Autodesk Inventor part; units mm, degrees
ref_plane "YZ Plane" through (0, 0, 0) normal (1, 0, 0) x (0, 1, 0)
ref_plane "XZ Plane" through (0, 0, 0) normal (0, 1, 0) x (-1, 0, 0)
ref_plane "XY Plane" through (0, 0, 0) normal (0, 0, 1) x (1, 0, 0)
sketch "Sketch1" plane through (0, 0, 0) normal (0, 0, 1) x (1, 0, 0)
  line L0 (-20.5, -12.375) -> (20.5, -12.375)
  line L1 (20.5, -12.375) -> (20.5, 12.375)
  line L2 (20.5, 12.375) -> (-20.5, 12.375)
  line L3 (-20.5, 12.375) -> (-20.5, -12.375)
  line L4 (-20.5, -12.375) -> (20.5, 12.375) construction
  line L5 (20.5, -12.375) -> (-20.5, 12.375) construction
  line L6 (-20.5, 12.375) -> (-25.5, 12.375) construction
  line L7 (20.5, 12.375) -> (25.5, 12.375) construction
  line L8 (20.5, -12.375) -> (25.5, -12.375) construction
  line L9 (25.5, -12.375) -> (25.5, -14.375) construction
  line L10 (-25.5, 12.375) -> (25.5, 12.375)
  line L11 (25.5, 12.375) -> (25.5, -14.375)
  line L12 (25.5, -14.375) -> (-25.5, -14.375)
  line L13 (-25.5, -14.375) -> (-25.5, 12.375)
  line L14 (-20.5, 12.375) -> (-13.5, 12.375)
  line L15 (20.5, 12.375) -> (13.5, 12.375)
  line L16 (13.5, 12.375) -> (13.5, 5.375) construction
  line L17 (-13.5, 12.375) -> (-13.5, 5.375) construction
  circle A0 centre (-13.5, 5.375) radius 7
  circle A1 centre (13.5, 5.375) radius 7
  point P0 (0, 0)
  point P1 (-20.5, 5.375)
  point P2 (20.5, 12.375)
  point P3 (20.5, 5.375)
  dimension "d0" = 41
  dimension "d3" = 24.75
  dimension "d4" = 5
  dimension "d5" = 5
  dimension "d6" = 5
  dimension "d7" = 2
  dimension "d8" = 7
  dimension "d9" = 7
  dimension "d10" = 7
  dimension "d11" = 7
extrude "Extrusion1" add sketch "Sketch1" along normal blind 7 contours L0 L1 L10 L11 L12 L13 L3 | L3 L2 A0 | A1 L2 L1
fillet "Fillet1" radius 7 2 edges at (-20.5, -12.375, 3.5) (20.5, -12.375, 3.5)
fillet "Fillet2" radius 4 2 edges at (-25.5, -14.375, 3.5) (25.5, -14.375, 3.5)
sketch "Sketch2" plane through (-25.5, 12.375, 0) normal (0, 1, 0) x (1, 0, 0)
  line L0 (0, 0) -> (2.5, 0) construction
  line L1 (12, 0) -> (0, 0) construction
  line L2 (2.5, 0) -> (2.5, -3.5) construction
  line L3 (12, -7) -> (0, -7) construction
  circle A0 centre (2.5, -3.5) radius 1.5
  line L4 (51, 0) -> (51, -7) construction
  line L5 (51, 0) -> (48.5, 0) construction
  line L6 (51, 0) -> (39, 0) construction
  line L7 (48.5, 0) -> (48.5, -3.5) construction
  circle A1 centre (48.5, -3.5) radius 1.5
  point P0 (25.5, 0)
  dimension "d16" = 2.5
  dimension "d17" = 3.5
  dimension "d18" = 3
  dimension "d19" = 2.5
  dimension "d20" = 3.5
  dimension "d21" = 3
extrude "Extrusion2" cut sketch "Sketch2" against normal blind 7
sketch "Sketch3" plane through (0, 0, 7) normal (0, 0, 1) x (1, 0, 0)
  arc A0 (-20.5, -5.375) -> (-13.5, -12.375) centre (-13.5, -5.375) ccw
  arc A1 (-25.5, -10.375) -> (-21.5, -14.375) centre (-21.5, -10.375) ccw
  line L0 (-13.5, -12.375) -> (-21.5, -12.375)
  line L1 (-21.5, -12.375) -> (-21.5, -14.375)
  line L2 (-21.5, -14.375) -> (-13.5, -14.375)
  line L3 (-13.5, -14.375) -> (-13.5, -12.375)
  line L4 (13.5, -12.375) -> (-13.5, -12.375)
  line L5 (-21.5, -14.375) -> (21.5, -14.375)
  line L6 (13.5, -12.375) -> (21.5, -12.375)
  line L7 (21.5, -12.375) -> (21.5, -14.375)
  line L8 (21.5, -14.375) -> (13.5, -14.375)
  line L9 (13.5, -14.375) -> (13.5, -12.375)
  line L10 (-13.5, -12.375) -> (13.5, -12.375)
  line L11 (13.5, -12.375) -> (13.5, -14.375)
  line L12 (13.5, -14.375) -> (-13.5, -14.375)
  line L13 (-13.5, -14.375) -> (-13.5, -12.375)
  point P0 (0, 0)
  dimension "d24" = 8
extrude "Extrusion3" add sketch "Sketch3" along normal blind 1
sketch "Sketch7" plane through (-21.5, -14.375, 7) normal (-1, 0, 0) x (0, 0, 1)
  line L0 (1, 0) -> (30, 0) construction
  line L1 (30, 0) -> (30, 4.5) construction
  line L2 (1, 2) -> (30, 4.5)
  line L3 (1, 0) -> (30, 2.25)
  line L4 (30, 4.5) -> (30, 6.5)
  line L5 (30, 6.5) -> (32, 6.5)
  line L6 (32, 6.5) -> (32, 2.4052)
  line L7 (32, 2.4052) -> (30, 2.25)
  line L8 (1, 0) -> (1, 2)
  point P0 (-7, 14.375)
  dimension "d42" = 29
  dimension "d43" = 4.5
  dimension "d44" = 2
  dimension "d45" = 2
extrude "Extrusion6" add sketch "Sketch7" against normal up to surface (43 mm away)
fillet "Fillet3" radius 8 1 edges at (0, -11.9698, 39)
fillet "Fillet4" radius 3 1 edges at (0, -9.875, 37)
sketch "Sketch8" plane through (-25.5, 12.375, 0) normal (0, 1, 0) x (1, 0, 0)
  line L0 (0, 0) -> (0, -7)
  line L1 (39, 0) -> (12, 0)
  line L2 (0, -7) -> (12, -7)
  line L3 (12, -7) -> (12, 0)
  line L4 (12, 0) -> (0, 0)
  line L5 (0, 0) -> (0, -7)
  line L6 (39, 0) -> (39, -7)
  line L7 (51, 0) -> (51, -7)
  line L8 (39, 0) -> (51, 0)
  line L9 (51, 0) -> (51, -7)
  line L10 (51, -7) -> (39, -7)
  line L11 (39, -7) -> (39, 0)
  circle A0 centre (48.5, -3.5) radius 1.5
  circle A1 centre (48.5, -3.5) radius 1.5
  circle A2 centre (2.5, -3.5) radius 1.5
  circle A3 centre (2.5, -3.5) radius 1.5
  line L12 (12, -7) -> (10, -7) construction
  line L13 (10, -7) -> (10, 0) construction
  line L14 (39, -7) -> (41, -7) construction
  line L15 (41, -7) -> (41, 0) construction
  arc A4 (10, -7) -> (10, 0) centre (7.9375, -3.5) ccw
  arc A5 (41, 0) -> (41, -7) centre (43.0625, -3.5) ccw
  point P0 (25.5, 0)
  point P1 (39, -3.5)
  point P2 (12, -3.5)
  dimension "d52" = 2
  dimension "d53" = 2
  dimension "d54" = 3
  dimension "d55" = 3
extrude "Extrusion7" cut sketch "Sketch8" against normal blind 1 contours L4 L3 A4 | A4 L3 L2 | L8 A5 L6 | A5 L10 L6
properties part number "SAW_clamp_sled"
Could you check a few things on this model? Use its own coordinates, in mm. A direction names the side the tool comes from. Round coordinates to 2 decimals unless told otherwise and drop trailing zeros. Write each loop counter-clockwise with the first axis right and the second up, starting at its lowest first coordinate (ties: lowest second). Pieces come first, ordered by that corner, then holes.
(1) Thinking about a two-plate mould opening in X: for faces 5 (the face through (-25.5, 1, 3)), 6 (the face through (-0.301, -13.443, 20.01)), 7 (the face through (24.3, -13.23, 3.55)), 8 (the face through (-20.5, 0, 3)), which applies, +X half, -X half, draft (parallel to the pull), parting line (faces both ways), or undercut?
Findings below:
face 5: -X half
face 6: draft
face 7: +X half
face 8: undercut
(2) If I drill on probe 1 along Z at (x, y) = (23, 8.75); probe 2 along X at (y, z) = (8, 3.5); probe 3 along X at (y, z) = (8.25, 3.5), over which ranges is the centre line in solid material (lowest first)?
Findings below:
probe 1: z = 0 to 2, 5 to 7
probe 2: x = -25.5 to -24.5, -21.5 to -19.99, 19.99 to 21.5, 24.5 to 25.5
probe 3: x = -25.5 to -24.5, -21.5 to -19.88, 19.88 to 21.5, 24.5 to 25.5
(3) Suppose I cut it at C-C on y = -7. Write out the boundary of the cut face in (x, z).
Findings below:
outline: (-25.5, 0) - (-20.31, 0) - (-20.31, 7) - (-25.5, 7) - close; (20.31, 0) - (25.5, 0) - (25.5, 7) - (20.31, 7) - close
(4) Which directions (+Z, -Z, +X, -X, +Y, -Y) give clear straight access to the entire face, cutting with the end or side of a thin tool? Please do faces 1 (the face through (20.5, 0, 3)), 2 (the face through (-18.504, -10.27, 3.549)), 3 (the face through (-23, 5.375, 3)), 4 (the face through (-24.36, -13.17, 3.55)).
Findings below:
face 1: +Z, -Z
face 2: -Z
face 3: +Y
face 4: +Z, -Z, -X, -Y
(5) For pin 1 (2 mm diameter, centred on x = 8, z = 37.5, fed in from +Y) (3 decimals); pin 2 (6 mm diameter, centred on x = 19, y = -1.5, fed in from +Z); pin 3 (4 mm diameter, centred on x = 9, z = 4.5, fed in from +Y) (3 decimals); pin 4 (4 mm diameter, centred on x = 13, z = 5.5, fed in from +Y) (3 decimals), each with a flat end and sliding along its axis, tell me the tip position at first contact or that it passes through.
Findings below:
pin 1: stops at y = -7.875
pin 2: stops at z = 7
pin 3: stops at y = -12.375
pin 4: stops at y = 12.375
(6) Suppose I cut it at A-A on y = 2. Write out the boundary of the cut face in (x, z).
Findings below:
outline: (-25.5, 0) - (-20.5, 0) - (-20.5, 7) - (-25.5, 7) - close; (20.5, 0) - (25.5, 0) - (25.5, 7) - (20.5, 7) - close
(7) Suppose I cut it at B-B on x = 0. Write out the boundary of the cut face in (y, z) (3 decimals).
Findings below:
outline: (-14.375, 0) - (-12.375, 0) - (-12.375, 8) - (-10.103, 34.356) arc R3 cw to (-7.875, 37) - (-7.875, 39) arc R8 ccw to (-12.485, 32.361) - (-14.375, 8) - close
(8) Suppose I cut it at D-D on z = 15. Write out the boundary of the cut face in (x, y), and give its area (3 significant figures).
Findings below:
outline: (-21.5, -13.83) - (21.5, -13.83) - (21.5, -11.77) - (-21.5, -11.77) - close
area: 88.6 mm2
